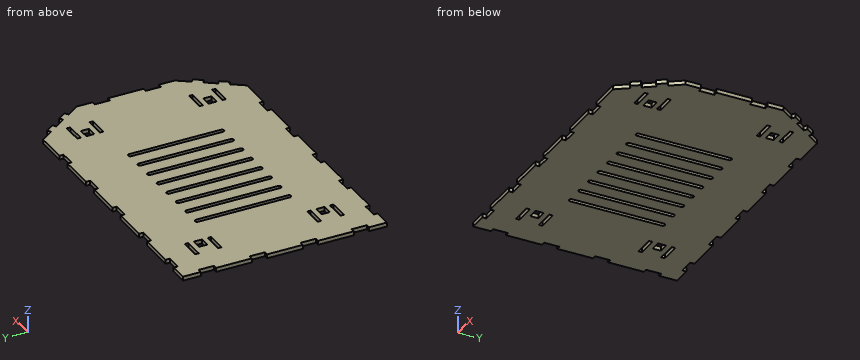
```python
from build123d import *

# Parameters (mm, degrees)
SKIZZE2_W                       = 300
SKIZZE2_H                       = 200
AUFSATZ_LINEAR_AUSTRAGEN1_DEPTH = 4
SKIZZE3_W                       = 15
SKIZZE3_H                       = 4
SCHNITT_LINEAR_AUSTRAGEN1_DEPTH = 4
LINEARES_MUSTER1_COUNT          = 6
LINEARES_MUSTER1_PITCH          = 50
SPIEGELN1_COPY_1_SKETCH_W       = 15
SPIEGELN1_COPY_1_SKETCH_H       = 4
SPIEGELN1_COPY_1_DEPTH          = 4
SPIEGELN1_COPY_2_SKETCH_W       = 15
SPIEGELN1_COPY_2_SKETCH_H       = 4
SPIEGELN1_COPY_2_DEPTH          = 4
SPIEGELN1_COPY_3_SKETCH_W       = 15
SPIEGELN1_COPY_3_SKETCH_H       = 4
SPIEGELN1_COPY_3_DEPTH          = 4
SPIEGELN1_COPY_4_SKETCH_W       = 15
SPIEGELN1_COPY_4_SKETCH_H       = 4
SPIEGELN1_COPY_4_DEPTH          = 4
SPIEGELN1_COPY_5_SKETCH_W       = 15
SPIEGELN1_COPY_5_SKETCH_H       = 4
SPIEGELN1_COPY_5_DEPTH          = 4
SKIZZE4_W                       = 4
SKIZZE4_H                       = 15
SCHNITT_LINEAR_AUSTRAGEN2_DEPTH = 4
LINEARES_MUSTER2_COUNT          = 4
LINEARES_MUSTER2_PITCH          = 50
SPIEGELN2_COPY_1_SKETCH_W       = 4
SPIEGELN2_COPY_1_SKETCH_H       = 15
SPIEGELN2_COPY_1_DEPTH          = 4
SPIEGELN2_COPY_2_SKETCH_W       = 4
SPIEGELN2_COPY_2_SKETCH_H       = 15
SPIEGELN2_COPY_2_DEPTH          = 4
SPIEGELN2_COPY_3_SKETCH_W       = 4
SPIEGELN2_COPY_3_SKETCH_H       = 15
SPIEGELN2_COPY_3_DEPTH          = 4
SKIZZE5_W                       = 19.7
SKIZZE5_H                       = 3.5
SCHNITT_LINEAR_AUSTRAGEN3_DEPTH = 4
SPIEGELN4_COPY_1_SKETCH_W       = 19.7
SPIEGELN4_COPY_1_SKETCH_H       = 3.5
SPIEGELN4_COPY_1_DEPTH          = 4
SCHNITT_LINEAR_AUSTRAGEN4_DEPTH = 4
SKIZZE8_W                       = 10
SKIZZE8_H                       = 8
SCHNITT_LINEAR_AUSTRAGEN5_DEPTH = 4
SPIEGELN7_COPY_1_SKETCH_W       = 10
SPIEGELN7_COPY_1_SKETCH_H       = 8
SPIEGELN7_COPY_1_DEPTH          = 4
SCHNITT_LINEAR_AUSTRAGEN6_DEPTH = 4
LINEARES_MUSTER3_COUNT          = 8
LINEARES_MUSTER3_PITCH          = 18
LINEARES_MUSTER3_COPY_1_DEPTH   = 4
LINEARES_MUSTER3_COPY_2_DEPTH   = 4
LINEARES_MUSTER3_COPY_3_DEPTH   = 4
LINEARES_MUSTER3_COPY_4_DEPTH   = 4
LINEARES_MUSTER3_COPY_5_DEPTH   = 4
LINEARES_MUSTER3_COPY_6_DEPTH   = 4
LINEARES_MUSTER3_COPY_7_DEPTH   = 4


with BuildPart() as part:
    # Skizze2 → Aufsatz-Linear austragen1 (new body)
    with BuildSketch(Plane.XY):
        with Locations((150, 100)):
            Rectangle(SKIZZE2_W, SKIZZE2_H)
    extrude(amount=AUFSATZ_LINEAR_AUSTRAGEN1_DEPTH)

    # Skizze3 → Schnitt-Linear austragen1 (cut)
    with BuildSketch(Plane.XY.offset(4)):
        with Locations((25, 198)):
            Rectangle(SKIZZE3_W, SKIZZE3_H)
    schnitt_linear_austragen1 = extrude(amount=-SCHNITT_LINEAR_AUSTRAGEN1_DEPTH, mode=Mode.SUBTRACT)

    # Lineares Muster1: Schnitt-Linear austragen1 ×6
    with Locations(*[(i * LINEARES_MUSTER1_PITCH, 0, 0) for i in range(1, LINEARES_MUSTER1_COUNT)]):
        add(schnitt_linear_austragen1, mode=Mode.SUBTRACT)

    # Spiegeln1: Schnitt-Linear austragen1 across plane
    add(schnitt_linear_austragen1.mirror(Plane.ZX.offset(100)), mode=Mode.SUBTRACT)

    # Spiegeln1 copy 1 sketch → Spiegeln1 copy 1 (cut)
    with BuildSketch(Plane(origin=(50, 200, 4), x_dir=(1, 0, 0), z_dir=(0, 0, 1))):
        with Locations((25, -198)):
            Rectangle(SPIEGELN1_COPY_1_SKETCH_W, SPIEGELN1_COPY_1_SKETCH_H)
    extrude(amount=-SPIEGELN1_COPY_1_DEPTH, mode=Mode.SUBTRACT)

    # Spiegeln1 copy 2 sketch → Spiegeln1 copy 2 (cut)
    with BuildSketch(Plane(origin=(100, 200, 4), x_dir=(1, 0, 0), z_dir=(0, 0, 1))):
        with Locations((25, -198)):
            Rectangle(SPIEGELN1_COPY_2_SKETCH_W, SPIEGELN1_COPY_2_SKETCH_H)
    extrude(amount=-SPIEGELN1_COPY_2_DEPTH, mode=Mode.SUBTRACT)

    # Spiegeln1 copy 3 sketch → Spiegeln1 copy 3 (cut)
    with BuildSketch(Plane(origin=(150, 200, 4), x_dir=(1, 0, 0), z_dir=(0, 0, 1))):
        with Locations((25, -198)):
            Rectangle(SPIEGELN1_COPY_3_SKETCH_W, SPIEGELN1_COPY_3_SKETCH_H)
    extrude(amount=-SPIEGELN1_COPY_3_DEPTH, mode=Mode.SUBTRACT)

    # Spiegeln1 copy 4 sketch → Spiegeln1 copy 4 (cut)
    with BuildSketch(Plane(origin=(200, 200, 4), x_dir=(1, 0, 0), z_dir=(0, 0, 1))):
        with Locations((25, -198)):
            Rectangle(SPIEGELN1_COPY_4_SKETCH_W, SPIEGELN1_COPY_4_SKETCH_H)
    extrude(amount=-SPIEGELN1_COPY_4_DEPTH, mode=Mode.SUBTRACT)

    # Spiegeln1 copy 5 sketch → Spiegeln1 copy 5 (cut)
    with BuildSketch(Plane(origin=(250, 200, 4), x_dir=(1, 0, 0), z_dir=(0, 0, 1))):
        with Locations((25, -198)):
            Rectangle(SPIEGELN1_COPY_5_SKETCH_W, SPIEGELN1_COPY_5_SKETCH_H)
    extrude(amount=-SPIEGELN1_COPY_5_DEPTH, mode=Mode.SUBTRACT)

    # Skizze4 → Schnitt-Linear austragen2 (cut)
    with BuildSketch(Plane.XY.offset(4)):
        with Locations((2, 175)):
            Rectangle(SKIZZE4_W, SKIZZE4_H)
    schnitt_linear_austragen2 = extrude(amount=-SCHNITT_LINEAR_AUSTRAGEN2_DEPTH, mode=Mode.SUBTRACT)

    # Lineares Muster2: Schnitt-Linear austragen2 ×4
    with Locations(*[(0, -i * LINEARES_MUSTER2_PITCH, 0) for i in range(1, LINEARES_MUSTER2_COUNT)]):
        add(schnitt_linear_austragen2, mode=Mode.SUBTRACT)

    # Spiegeln2: Schnitt-Linear austragen2 across plane
    add(schnitt_linear_austragen2.mirror(Plane.ZY.offset(-150)), mode=Mode.SUBTRACT)

    # Spiegeln2 copy 1 sketch → Spiegeln2 copy 1 (cut)
    with BuildSketch(Plane(origin=(300, -50, 4), x_dir=(-1, 0, 0), z_dir=(0, 0, 1))):
        with Locations((2, -175)):
            Rectangle(SPIEGELN2_COPY_1_SKETCH_W, SPIEGELN2_COPY_1_SKETCH_H)
    extrude(amount=-SPIEGELN2_COPY_1_DEPTH, mode=Mode.SUBTRACT)

    # Spiegeln2 copy 2 sketch → Spiegeln2 copy 2 (cut)
    with BuildSketch(Plane(origin=(300, -100, 4), x_dir=(-1, 0, 0), z_dir=(0, 0, 1))):
        with Locations((2, -175)):
            Rectangle(SPIEGELN2_COPY_2_SKETCH_W, SPIEGELN2_COPY_2_SKETCH_H)
    extrude(amount=-SPIEGELN2_COPY_2_DEPTH, mode=Mode.SUBTRACT)

    # Spiegeln2 copy 3 sketch → Spiegeln2 copy 3 (cut)
    with BuildSketch(Plane(origin=(300, -150, 4), x_dir=(-1, 0, 0), z_dir=(0, 0, 1))):
        with Locations((2, -175)):
            Rectangle(SPIEGELN2_COPY_3_SKETCH_W, SPIEGELN2_COPY_3_SKETCH_H)
    extrude(amount=-SPIEGELN2_COPY_3_DEPTH, mode=Mode.SUBTRACT)

    # Skizze5 → Schnitt-Linear austragen3 (cut)
    with BuildSketch(Plane.XY.offset(4)):
        with Locations((38.85, 171.15)):
            Rectangle(SKIZZE5_W, SKIZZE5_H)
        with Locations((38.85, 148.85)):
            Rectangle(SKIZZE5_W, SKIZZE5_H)
    schnitt_linear_austragen3 = extrude(amount=-SCHNITT_LINEAR_AUSTRAGEN3_DEPTH, mode=Mode.SUBTRACT)

    # Spiegeln3: Schnitt-Linear austragen3 across plane
    add(schnitt_linear_austragen3.mirror(Plane.ZY.offset(-150)), mode=Mode.SUBTRACT)

    # Spiegeln4: Schnitt-Linear austragen3 across plane
    add(schnitt_linear_austragen3.mirror(Plane.ZX.offset(100)), mode=Mode.SUBTRACT)

    # Spiegeln4 copy 1 sketch → Spiegeln4 copy 1 (cut)
    with BuildSketch(Plane(origin=(300, 200, 4), x_dir=(-1, 0, 0), z_dir=(0, 0, 1))):
        with Locations((38.85, 171.15)):
            Rectangle(SPIEGELN4_COPY_1_SKETCH_W, SPIEGELN4_COPY_1_SKETCH_H)
        with Locations((38.85, 148.85)):
            Rectangle(SPIEGELN4_COPY_1_SKETCH_W, SPIEGELN4_COPY_1_SKETCH_H)
    extrude(amount=-SPIEGELN4_COPY_1_DEPTH, mode=Mode.SUBTRACT)

    # Skizze7 → Schnitt-Linear austragen4 (cut)
    with BuildSketch(Plane.XY.offset(4)):
        Polygon((263.589208013, 0), (272.330592807, 12.483991269), (275.607200984, 10.189685524), (281.342965347, 18.381205967), (278.06635717, 20.675511712), (285.522850843, 31.324488288), (288.79945902, 29.030182542), (294.535223383, 37.221702985), (291.258615206, 39.516008731), (300, 52), (300, 0), align=None)
    schnitt_linear_austragen4 = extrude(amount=-SCHNITT_LINEAR_AUSTRAGEN4_DEPTH, mode=Mode.SUBTRACT)

    # Spiegeln5: Schnitt-Linear austragen4 across plane
    add(schnitt_linear_austragen4.mirror(Plane.ZX.offset(100)), mode=Mode.SUBTRACT)

    # Skizze8 → Schnitt-Linear austragen5 (cut)
    with BuildSketch(Plane.XY.offset(4)):
        with Locations((256.3, 160)):
            Rectangle(SKIZZE8_W, SKIZZE8_H)
    schnitt_linear_austragen5 = extrude(amount=-SCHNITT_LINEAR_AUSTRAGEN5_DEPTH, mode=Mode.SUBTRACT)

    # Spiegeln6: Schnitt-Linear austragen5 across plane
    add(schnitt_linear_austragen5.mirror(Plane.ZY.offset(-150)), mode=Mode.SUBTRACT)

    # Spiegeln7: Schnitt-Linear austragen5 across plane
    add(schnitt_linear_austragen5.mirror(Plane.ZX.offset(100)), mode=Mode.SUBTRACT)

    # Spiegeln7 copy 1 sketch → Spiegeln7 copy 1 (cut)
    with BuildSketch(Plane(origin=(300, 200, 4), x_dir=(-1, 0, 0), z_dir=(0, 0, 1))):
        with Locations((256.3, 160)):
            Rectangle(SPIEGELN7_COPY_1_SKETCH_W, SPIEGELN7_COPY_1_SKETCH_H)
    extrude(amount=-SPIEGELN7_COPY_1_DEPTH, mode=Mode.SUBTRACT)

    # Skizze9 → Schnitt-Linear austragen6 (cut)
    with BuildSketch(Plane.XY.offset(4)):
        with BuildLine():
            Line((207, 100), (203, 100))
            Line((203, 100), (203, 145))
            ThreePointArc((203, 145), (205, 147), (207, 145))
            Line((207, 145), (207, 100))
        make_face()
    schnitt_linear_austragen6 = extrude(amount=-SCHNITT_LINEAR_AUSTRAGEN6_DEPTH, mode=Mode.SUBTRACT)

    # Spiegeln8: Schnitt-Linear austragen6 across plane
    add(schnitt_linear_austragen6.mirror(Plane.ZX.offset(100)), mode=Mode.SUBTRACT)

    # Lineares Muster3: Schnitt-Linear austragen6 ×8
    with Locations(*[(-i * LINEARES_MUSTER3_PITCH, 0, 0) for i in range(1, LINEARES_MUSTER3_COUNT)]):
        add(schnitt_linear_austragen6, mode=Mode.SUBTRACT)

    # Lineares Muster3 copy 1 sketch → Lineares Muster3 copy 1 (cut)
    with BuildSketch(Plane(origin=(-18, 200, 4), x_dir=(1, 0, 0), z_dir=(0, 0, 1))):
        with BuildLine():
            Line((207, -100), (203, -100))
            Line((203, -100), (203, -145))
            ThreePointArc((203, -145), (205, -147), (207, -145))
            Line((207, -145), (207, -100))
        make_face()
    extrude(amount=-LINEARES_MUSTER3_COPY_1_DEPTH, mode=Mode.SUBTRACT)

    # Lineares Muster3 copy 2 sketch → Lineares Muster3 copy 2 (cut)
    with BuildSketch(Plane(origin=(-36, 200, 4), x_dir=(1, 0, 0), z_dir=(0, 0, 1))):
        with BuildLine():
            Line((207, -100), (203, -100))
            Line((203, -100), (203, -145))
            ThreePointArc((203, -145), (205, -147), (207, -145))
            Line((207, -145), (207, -100))
        make_face()
    extrude(amount=-LINEARES_MUSTER3_COPY_2_DEPTH, mode=Mode.SUBTRACT)

    # Lineares Muster3 copy 3 sketch → Lineares Muster3 copy 3 (cut)
    with BuildSketch(Plane(origin=(-54, 200, 4), x_dir=(1, 0, 0), z_dir=(0, 0, 1))):
        with BuildLine():
            Line((207, -100), (203, -100))
            Line((203, -100), (203, -145))
            ThreePointArc((203, -145), (205, -147), (207, -145))
            Line((207, -145), (207, -100))
        make_face()
    extrude(amount=-LINEARES_MUSTER3_COPY_3_DEPTH, mode=Mode.SUBTRACT)

    # Lineares Muster3 copy 4 sketch → Lineares Muster3 copy 4 (cut)
    with BuildSketch(Plane(origin=(-72, 200, 4), x_dir=(1, 0, 0), z_dir=(0, 0, 1))):
        with BuildLine():
            Line((207, -100), (203, -100))
            Line((203, -100), (203, -145))
            ThreePointArc((203, -145), (205, -147), (207, -145))
            Line((207, -145), (207, -100))
        make_face()
    extrude(amount=-LINEARES_MUSTER3_COPY_4_DEPTH, mode=Mode.SUBTRACT)

    # Lineares Muster3 copy 5 sketch → Lineares Muster3 copy 5 (cut)
    with BuildSketch(Plane(origin=(-90, 200, 4), x_dir=(1, 0, 0), z_dir=(0, 0, 1))):
        with BuildLine():
            Line((207, -100), (203, -100))
            Line((203, -100), (203, -145))
            ThreePointArc((203, -145), (205, -147), (207, -145))
            Line((207, -145), (207, -100))
        make_face()
    extrude(amount=-LINEARES_MUSTER3_COPY_5_DEPTH, mode=Mode.SUBTRACT)

    # Lineares Muster3 copy 6 sketch → Lineares Muster3 copy 6 (cut)
    with BuildSketch(Plane(origin=(-108, 200, 4), x_dir=(1, 0, 0), z_dir=(0, 0, 1))):
        with BuildLine():
            Line((207, -100), (203, -100))
            Line((203, -100), (203, -145))
            ThreePointArc((203, -145), (205, -147), (207, -145))
            Line((207, -145), (207, -100))
        make_face()
    extrude(amount=-LINEARES_MUSTER3_COPY_6_DEPTH, mode=Mode.SUBTRACT)

    # Lineares Muster3 copy 7 sketch → Lineares Muster3 copy 7 (cut)
    with BuildSketch(Plane(origin=(-126, 200, 4), x_dir=(1, 0, 0), z_dir=(0, 0, 1))):
        with BuildLine():
            Line((207, -100), (203, -100))
            Line((203, -100), (203, -145))
            ThreePointArc((203, -145), (205, -147), (207, -145))
            Line((207, -145), (207, -100))
        make_face()
    extrude(amount=-LINEARES_MUSTER3_COPY_7_DEPTH, mode=Mode.SUBTRACT)


solid = part.part
```
Here's how the part is built. I have some questions about the finished solid (model axes, mm). Round coordinates to 2 decimals unless told otherwise and drop trailing zeros. Use CSV: the item, a comma, the result in double quotes.
1) I need wall thicknesses on line 1 along X through (y, z) = (171.5, 1.65); line 2 along X through (y, z) = (150, 3.7); line 3 along Y through (x, z) = (186, 3.6). Which ranges of each line are inside material? Lowest first, please. Write a range as [from, to].
Taken from the geometry:
line 1,"[4, 29], [48.7, 251.3], [271, 283.55]"
line 2,"[0, 29], [48.7, 251.3], [271, 298.6]"
line 3,"[0, 53.27], [146.73, 200]"
2) I'm going to push flat-ended pins straight in: P1, Ø1.5, axis at y = 76, z = 3.5, coming from the -X side; P2, Ø5, axis at x = 170, y = 123, coming from the +Z side; P3, Ø1.2, axis at x = 178, z = 1.5, coming from the +Y side. Where does each tip first touch, or does it pass through?
Taken from the geometry:
P1,"x = 4"
P2,"z = 4"
P3,"y = 196"
3) I want a section at A-A (y = 122.5). Count the separate pieces of the cut face and the enclosed holes in it, then the cut area to 3 significant figures.
Taken from the geometry:
separate pieces,"9"
enclosed holes,"0"
area,"1,040 mm^2"
